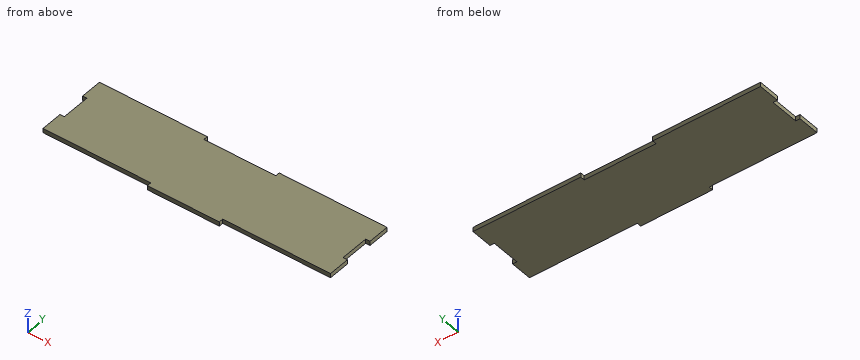
Autodesk Inventor part; units mm, degrees
ref_plane "YZ Plane" through (0, 0, 0) normal (1, 0, 0) x (0, 1, 0)
ref_plane "XZ Plane" through (0, 0, 0) normal (0, 1, 0) x (-1, 0, 0)
ref_plane "XY Plane" through (0, 0, 0) normal (0, 0, 1) x (1, 0, 0)
sketch "스케치1" plane through (0, 0, 0) normal (0, 0, 1) x (1, 0, 0)
  line L0 (-100, -25) -> (100, -25)
  line L1 (100, -25) -> (100, 25)
  line L2 (100, 25) -> (-100, 25)
  line L3 (-100, 25) -> (-100, -25)
  line L4 (-100, -25) -> (100, 25) construction
  line L5 (100, -25) -> (-100, 25) construction
  line L6 (-25, 22) -> (25, 22)
  line L7 (25, 22) -> (25, 28)
  line L8 (25, 28) -> (-25, 28)
  line L9 (-25, 28) -> (-25, 22)
  line L10 (-25, 22) -> (25, 28) construction
  line L11 (25, 22) -> (-25, 28) construction
  line L12 (-103, -10) -> (-97, -10)
  line L13 (-97, -10) -> (-97, 10)
  line L14 (-97, 10) -> (-103, 10)
  line L15 (-103, 10) -> (-103, -10)
  line L16 (-103, -10) -> (-97, 10) construction
  line L17 (-97, -10) -> (-103, 10) construction
  line L18 (97, -10) -> (103, -10)
  line L19 (103, -10) -> (103, 10)
  line L20 (103, 10) -> (97, 10)
  line L21 (97, 10) -> (97, -10)
  line L22 (97, -10) -> (103, 10) construction
  line L23 (103, -10) -> (97, 10) construction
  point P0 (0, 0)
  point P1 (0, 25)
  point P2 (-100, 0)
  point P3 (100, 0)
  point P4 (-100, -10)
  point P5 (100, -10)
  point P6 (100, 10)
  point P7 (25, 25)
  point P8 (-25, 25)
  point P9 (-100, 10)
  dimension "d0" = 50
  dimension "d1" = 200
  dimension "d2" = 50
  dimension "d3" = 3
  dimension "d4" = 20
  dimension "d5" = 20
  dimension "d6" = 3
  dimension "d7" = 3
extrude "돌출1" add sketch "스케치1" along normal blind 3 contours L3 L12 L13 L14 L2 L9 L6 L7 L1 L20 L21 L18 L0
sketch "스케치2" plane through (0, 0, 3) normal (0, 0, 1) x (1, 0, 0)
  line L0 (-25, -22) -> (25, -22)
  line L1 (25, -22) -> (25, -28)
  line L2 (25, -28) -> (-25, -28)
  line L3 (-25, -28) -> (-25, -22)
  line L4 (-100, -25) -> (100, -25)
  line L5 (-25, -22) -> (25, -28) construction
  line L6 (25, -22) -> (-25, -28) construction
  point P0 (0, 0)
  point P1 (0, -25)
  point P2 (25, -25)
  point P3 (-25, -25)
  dimension "d10" = 50
  dimension "d11" = 3
extrude "돌출2" add sketch "스케치2" against normal blind 3 contours L4 L1 L2 L3
sketch "스케치3" plane through (0, 0, 3) normal (0, 0, 1) x (1, 0, 0)
  point P0 (0, 0)
sketch "스케치4" plane through (0, 0, 3) normal (0, 0, 1) x (1, 0, 0)
  point P0 (0, 0)
properties part number "본체 겉면 레이저 옆판 수정"
For this review, take the finished solid that the model builds, in its own axes (mm). Give positions to 0.01 mm unless a question says otherwise; leave off trailing zeros. Order: outer loops, then holes, each group sorted by start corner. A loop starts at its lowest first (then second) coordinate and runs counter-clockwise, first axis right, second up. Notation, with made-up numbers: (18, 53.25) - (26, 53.25) arc R26 ccw to (26, 82.25) - close; hole circle Ø10 at (68.25, 48.25). An arc over 180 degrees is marked (long way). Answer as a JSON object with one key per item and string values. Group by question number.
Item 1: Clearance check with flat-ended pins moving along their axes: pin 1 Ø1.5 at (x, z) = (74.5, 1) entering from -Y; pin 2 Ø1.5 at (y, z) = (4, 1) entering from -X; pin 3 Ø1.5 at (y, z) = (-1.5, 1) entering from +X. State where each tip first meets the part, or that it passes through.
Item 2: Take a section at B-B on y = -5. Give the boundary of the cut face in (x, z).
Item 3: Wall thickness on line 1 along Y through (x, z) = (-89.5, 2); line 2 along Y through (x, z) = (21, 2.35); line 3 along X through (y, z) = (4, 0.1): over which ranges is each line inside the solid? List them lowest first.
Item 4: Take a section at C-C on x = 67. Give the boundary of the cut face in (y, z), and give its area (3 significant figures).
Item 5: Take a section at A-A on z = 2.3. Give the boundary of the cut face in (x, y).
Reported:
{
 "1": {"pin 1": "y = -25", "pin 2": "x = -97", "pin 3": "x = 97"},
 "2": {"outline": "(-97, 0) - (97, 0) - (97, 3) - (-97, 3) - close"},
 "3": {"line 1": "-25 to 25", "line 2": "-28 to 22", "line 3": "-97 to 97"},
 "4": {"outline": "(-25, 0) - (25, 0) - (25, 3) - (-25, 3) - close", "area": "150 mm^2"},
 "5": {"outline": "(-100, -25) - (-25, -25) - (-25, -28) - (25, -28) - (25, -25) - (100, -25) - (100, -10) - (97, -10) - (97, 10) - (100, 10) - (100, 25) - (25, 25) - (25, 22) - (-25, 22) - (-25, 25) - (-100, 25) - (-100, 10) - (-97, 10) - (-97, -10) - (-100, -10) - close"}
}
